For this review, take the finished solid that the model builds, in its own axes (mm). Give positions to 0.01 mm unless a question says otherwise; leave off trailing zeros. Write each loop counter-clockwise with the first axis right and the second up, starting at its lowest first coordinate (ties: lowest second). Pieces come first, ordered by that corner, then holes. Notation, with made-up numbers: M -12.75,-7.5 L 35.25,-7.5 A19 ccw 35.25,20.5 Z; hole C 67.5,-25 d6. An arc over 180 degrees is marked long. Use one line per item in the form item = value. Start each with the question number.
Q1. Consider section A-A on y = -0.1. Write out the cut boundary in (x, z) (3 decimals), and give its area (3 significant figures).
Q2. Clearance check with flat-ended pins moving along their axes: pin 1 Ø0.5 at (x, z) = (0, 4) entering from -Y (3 decimals); pin 2 Ø0.5 at (y, z) = (0, -3) entering from -X (3 decimals); pin 3 Ø0.7 at (y, z) = (0, 3.5) entering from +X (3 decimals). State where each tip first meets the part, or that it passes through.
Q3. For probe 1 along Z at (x, y) = (0, -0.8); probe 2 along X at (y, z) = (-0.15, -3.25) (3 decimals), list the stretches that pass through material, from the lowest coordinate up. Write a range as [from, to].
Q4. Consider section B-B on z = 1.5. Write out the cut boundary in (x, y), and give its area (3 significant figures).
Q5. Consider section D-D on z = 2.75. Write out the cut boundary in (x, y) (3 decimals).
Q6. Consider section C-C on x = -0.6. Write out the cut boundary in (y, z).
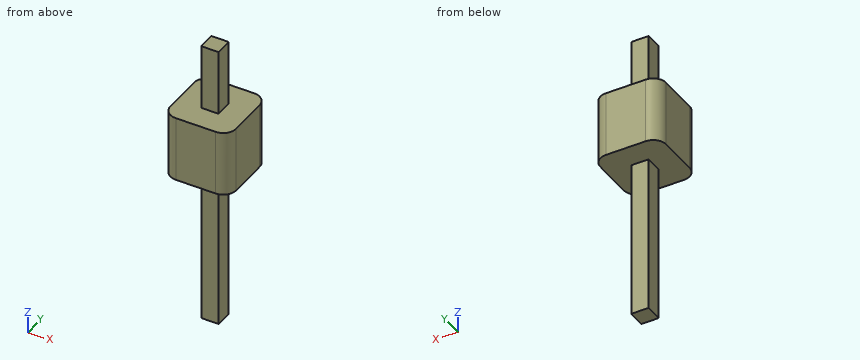
```python
from build123d import *

# Parameters (mm, degrees)
SKETCH_1_W      = 2.54
SKETCH_1_H      = 2.54
EXTRUDE_1_DEPTH = 2.54
SKETCH_2_W      = 0.67
SKETCH_2_H      = 0.67
FILLET_1_R      = 0.5


with BuildPart() as part:
    # 草图1 → 拉伸1 (new body)
    with BuildSketch(Plane.XY):
        Rectangle(SKETCH_1_W, SKETCH_1_H)
    extrude(amount=EXTRUDE_1_DEPTH)

    # 扫描1: sweep along a path in 草图3
    with BuildLine(Plane(origin=(0, 0, 0), x_dir=(0, 0, -1), z_dir=(1, 0, 0))) as sweep_1_path:
        Line((6.12, -0.01), (-5.08, -0.01))
    # 草图2 → 扫描1 (sweep)
    with BuildSketch(Plane(origin=(0, 0, 5.08), x_dir=(-1, 0, 0), z_dir=(0, 0, -1))):
        Rectangle(SKETCH_2_W, SKETCH_2_H)
    sweep(path=sweep_1_path.line)

    # 圆角1
    fillet_1_edges = [part.edges().sort_by_distance(p)[0] for p in [
        (-1.27, 1.27, 1.27),
        (1.27, 1.27, 1.27),
        (1.27, -1.27, 1.27),
        (-1.27, -1.27, 1.27),
    ]]
    fillet(fillet_1_edges, radius=FILLET_1_R)


solid = part.part
```
Working result:
q1.outline = M -1.27,0 L -0.335,0 L -0.335,-6.12 L 0.335,-6.12 L 0.335,0 L 1.27,0 L 1.27,2.54 L 0.335,2.54 L 0.335,5.08 L -0.335,5.08 L -0.335,2.54 L -1.27,2.54 Z
q1.area = 12.3 mm²
q2.pin_1 = -0.335
q2.pin_2 = -0.335
q2.pin_3 = 0.335
q3.probe_1 = [0, 2.54]
q3.probe_2 = [-0.335, 0.335]
q4.outline = M -1.27,-0.77 A0.5 ccw -0.77,-1.27 L 0.77,-1.27 A0.5 ccw 1.27,-0.77 L 1.27,0.77 A0.5 ccw 0.77,1.27 L -0.77,1.27 A0.5 ccw -1.27,0.77 Z
q4.area = 6.24 mm²
q5.outline = M -0.335,-0.335 L 0.335,-0.335 L 0.335,0.335 L -0.335,0.335 Z
q6.outline = M -1.27,0 L 1.27,0 L 1.27,2.54 L -1.27,2.54 Z
